Verification items for the finished model (mm, model axes). A direction names the side the tool comes from. Round coordinates to 2 decimals unless told otherwise and drop trailing zeros. Write each loop counter-clockwise with the first axis right and the second up, starting at its lowest first coordinate (ties: lowest second). Pieces come first, ordered by that corner, then holes. Notation, with made-up numbers: (88.5, 33) - (120.5, 33) arc R8 cw to (120.5, 42) - close; hole circle Ø7 at (-30, 6). An arc over 180 degrees is marked (long way). Answer as a JSON object with one key per item and string values.
```python
from build123d import *

# Parameters (mm, degrees)
SKETCH1_R                = 3.175
SKETCH1_W                = 3.2258
SKETCH1_H                = 6.35
BOSS_EXTRUDE1_DEPTH      = 3.175
ADD_BODY_AT_BOTTOM_DEPTH = 3.175
CUT_EXTRUDE1_DEPTH       = 4.175


with BuildPart() as part:
    # Sketch1 → Boss-Extrude1 (new body)
    with BuildSketch(Plane(origin=(0, 0, 0), x_dir=(0, 0, -1), z_dir=(1, 0, 0))):
        Polygon((-6.985, 7.62), (6.985, 7.62), (6.985, -22.606), (-33.782, -22.606), (-33.782, -16.256), (-37.0078, -16.256), (-37.0078, -9.906), (-33.782, -9.906), (-33.782, -7.366), (-27.94, -7.366), (-27.94, -16.764), (-18.796, -16.764), (-18.796, -7.366), (-6.985, -7.366), align=None)
        Circle(SKETCH1_R, mode=Mode.SUBTRACT)
        with Locations((-10.5791, -14.351)):
            Rectangle(SKETCH1_W, SKETCH1_H, mode=Mode.SUBTRACT)
    extrude(amount=BOSS_EXTRUDE1_DEPTH)

    # Sketch2 → add body at bottom (add)
    with BuildSketch(Plane.ZY):
        with BuildLine():
            Line((23.368, -22.606), (15.748, -22.606))
            ThreePointArc((15.748, -22.606), (23.368, -24.321629486), (30.988, -22.606))
            Line((30.988, -22.606), (23.368, -22.606))
        make_face()
    extrude(amount=-ADD_BODY_AT_BOTTOM_DEPTH)

    # Sketch3 → Cut-Extrude1 (cut, through all)
    with BuildSketch(Plane.ZY):
        Polygon((30.861, -7.366), (27.94, -12.065), (27.94, -7.366), align=None)
        with BuildLine():
            Line((-6.985, -22.606), (-0.635, -22.606))
            ThreePointArc((-0.635, -22.606), (-4.50973023, -18.660807307), (-6.985, -13.716))
            Line((-6.985, -13.716), (-6.985, -22.606))
        make_face()
    extrude(amount=-CUT_EXTRUDE1_DEPTH, mode=Mode.SUBTRACT)


solid = part.part
```
1. Cross-section at D-D (z = 5.5). Record the boundary of the cut face in (x, y) (3 decimals).
Completed:
{"outline": "(0, -22.606) - (3.175, -22.606) - (3.175, 7.62) - (0, 7.62) - close"}
2. Cross-section at A-A (z = 10). Record the boundary of the cut face in (x, y) (3 decimals), plus the area to 3 significant figures.
Completed:
{"outline": "(0, -22.606) - (3.175, -22.606) - (3.175, -17.526) - (0, -17.526) - close; (0, -11.176) - (3.175, -11.176) - (3.175, -7.366) - (0, -7.366) - close", "area": "28.2 mm^2"}
3. Go/stop test with flat-tipped pins: pin 1 (1.6 mm diameter, centred on x = 1.5, z = 10, fed in from -Y); pin 2 (4 mm diameter, centred on y = -12.5, z = 24.5, fed in from +X); pin 3 (1 mm diameter, centred on y = -15.5, z = 0, fed in from -X); pin 4 (1.6 mm diameter, centred on x = 2, z = 36, fed in from +Y). Record where each tip stops, or that it passes through.
Completed:
{"pin 1": "stops at y = -22.61", "pin 2": "passes through", "pin 3": "stops at x = 0", "pin 4": "stops at y = -9.91"}
4. Mould release check, pull along Y, two halves, no side actions. Record for faces 1 (the face through (1.565, -18.724, -4.464)), 2 (the face through (2, -17.526, 11)), 3 (the face through (2, 0, 6.985)): released by +Y, released by -Y, zero draft, split by the parting line, or undercut.
Completed:
{"face 1": "released by -Y", "face 2": "undercut", "face 3": "zero draft"}
5. Cross-section at B-B (y = 0). Record the boundary of the cut face in (x, z) (3 decimals), plus the area to 3 significant figures.
Completed:
{"outline": "(0, -6.985) - (3.175, -6.985) - (3.175, -3.175) - (0, -3.175) - close; (0, 3.175) - (3.175, 3.175) - (3.175, 6.985) - (0, 6.985) - close", "area": "24.2 mm^2"}
6. Material ranges on probe 1 along Y at (x, z) = (2.1, 0) (3 decimals); probe 2 along Z at (x, y) = (0.25, -4) (3 decimals); probe 3 along Y at (x, z) = (1.15, 12), recorded low to high. Write a range as from..to.
Completed:
{"probe 1": "y = -22.606..-3.175, 3.175..7.62", "probe 2": "z = -6.985..6.985", "probe 3": "y = -22.61..-17.53, -11.18..-7.37"}
7. Cross-section at C-C (x = 1.85). Record the boundary of the cut face in (y, z) (3 decimals).
Completed:
{"outline": "(-22.606, -0.635) arc R17.78 ccw to (-13.716, -6.985) - (7.62, -6.985) - (7.62, 6.985) - (-7.366, 6.985) - (-7.366, 18.796) - (-16.764, 18.796) - (-16.764, 27.94) - (-12.065, 27.94) - (-7.366, 30.861) - (-7.366, 33.782) - (-9.906, 33.782) - (-9.906, 37.008) - (-16.256, 37.008) - (-16.256, 33.782) - (-22.606, 33.782) - (-22.606, 30.988) arc R17.78 ccw to (-22.606, 15.748) - close; hole (-17.526, 8.966) - (-11.176, 8.966) - (-11.176, 12.192) - (-17.526, 12.192) - close; hole circle Ø6.35 at (0, 0)"}
8. Access from +Z, -Z, +X, -X, +Y, -Y to the whole of each face (thin tool, end or side, straight path). Record for faces 4 (the face through (2, -14, 27.94)), 5 (the face through (2, -9, 33.782)), 6 (the face through (2, -14, 8.966)), 7 (the face through (2, -16.256, 35)).
Completed:
{"face 4": "+X, -X, +Y", "face 5": "+Z, +X, -X, +Y", "face 6": "+X, -X", "face 7": "+Z, +X, -X, -Y"}
